Model file for the job. Use its own axes, mm. A direction names the side the tool comes from. Round coordinates to 2 decimals unless told otherwise and drop trailing zeros. Loops run counter-clockwise (first coordinate to the right, second up) from the corner with the lowest first, then second, coordinate; pieces in that order, holes last. Notation, with made-up numbers: (-9, 87.25) -> (14, 87.25) arc R19 ccw to (14, 98.25) -> close; hole circle Ø6 at (59.25, -17). An arc over 180 degrees is marked (long way). Use a Markdown table: item, result.
from build123d import *

# Parameters (mm, degrees)
BOSS_EXTRU_1_DEPTH      = 132
ESQUISSE2_W             = 78
ESQUISSE2_H             = 14.57
ENL_V_MAT_EXTRU_1_DEPTH = 132
ESQUISSE3_W             = 4.94012132
ESQUISSE3_H             = 29.556292602
ENL_V_MAT_EXTRU_2_DEPTH = 4
ESQUISSE4_R             = 1.3
ENL_V_MAT_EXTRU_3_DEPTH = 18
ESQUISSE6_R             = 2.9
ENL_V_MAT_EXTRU_5_DEPTH = 3


with BuildPart() as part:
    # Esquisse1 → Boss.-Extru.1 (new body)
    with BuildSketch(Plane.XY):
        with BuildLine():
            Line((-12.560062385, 0), (-18.560062385, 0))
            Line((-18.560062385, 0), (-18.560062385, 18))
            Line((-18.560062385, 18), (18.560062385, 18))
            Line((18.560062385, 18), (18.560062385, 0))
            Line((18.560062385, 0), (12.560062385, 0))
            ThreePointArc((12.560062385, 0), (0, 12.560062385), (-12.560062385, 0))
        make_face()
    extrude(amount=BOSS_EXTRU_1_DEPTH)

    # Esquisse2 → Enlèv. mat.-Extru.1 (cut)
    with BuildSketch(Plane.ZY.offset(18.560062385)):
        with Locations((66, 7.285)):
            Rectangle(ESQUISSE2_W, ESQUISSE2_H)
    extrude(amount=-ENL_V_MAT_EXTRU_1_DEPTH, mode=Mode.SUBTRACT)

    # Esquisse3 → Enlèv. mat.-Extru.2 (cut)
    with BuildSketch(Plane.XZ.offset(-14.57)):
        with Locations((0, 66)):
            Rectangle(ESQUISSE3_W, ESQUISSE3_H)
    extrude(amount=-ENL_V_MAT_EXTRU_2_DEPTH, mode=Mode.SUBTRACT)

    # Esquisse4 → Enlèv. mat.-Extru.3 (cut)
    with BuildSketch(Plane(origin=(0, 18, 0), x_dir=(1, 0, 0), z_dir=(0, 1, 0))):
        with Locations((15.560062385, -3)):
            Circle(ESQUISSE4_R)
        with Locations((15.560062385, -24)):
            Circle(ESQUISSE4_R)
        with Locations((-15.560062385, -3)):
            Circle(ESQUISSE4_R)
        with Locations((-15.560062385, -24)):
            Circle(ESQUISSE4_R)
        with Locations((-15.560062385, -108)):
            Circle(ESQUISSE4_R)
        with Locations((-15.560062385, -129)):
            Circle(ESQUISSE4_R)
        with Locations((15.560062385, -108)):
            Circle(ESQUISSE4_R)
        with Locations((15.560062385, -129)):
            Circle(ESQUISSE4_R)
    extrude(amount=-ENL_V_MAT_EXTRU_3_DEPTH, mode=Mode.SUBTRACT)

    # Esquisse6 → Enlèv. mat.-Extru.5 (cut)
    with BuildSketch(Plane(origin=(0, 18, 0), x_dir=(1, 0, 0), z_dir=(0, 1, 0))):
        with Locations((15.560062385, -3)):
            Circle(ESQUISSE6_R)
        with Locations((15.560062385, -24)):
            Circle(ESQUISSE6_R)
        with Locations((-15.560062385, -3)):
            Circle(ESQUISSE6_R)
        with Locations((-15.560062385, -24)):
            Circle(ESQUISSE6_R)
        with Locations((-15.560062385, -108)):
            Circle(ESQUISSE6_R)
        with Locations((-15.560062385, -129)):
            Circle(ESQUISSE6_R)
        with Locations((15.560062385, -108)):
            Circle(ESQUISSE6_R)
        with Locations((15.560062385, -129)):
            Circle(ESQUISSE6_R)
    extrude(amount=-ENL_V_MAT_EXTRU_5_DEPTH, mode=Mode.SUBTRACT)


solid = part.part
Q1. Flat gauge pins, fed straight in: pin 1 (1.6 mm diameter, centred on x = 15.56, z = 24, fed in from +Y); pin 2 (3 mm diameter, centred on x = -15.5, z = 2, fed in from +Y). Where does each tip first touch, or does it go through?
Results list:
| item | result |
|---|---|
| pin 1 | passes through |
| pin 2 | stops at y = 15 |
Q2. Tool access for faces 1 (the face through (-4.4, 12, 105)), 2 (the face through (-16.19, 16.52, 110.83)), 3 (the face through (2.47, 16, 66)): list every direction of +Z, -Z, +X, -X, +Y, -Y with a clear straight run to the whole face (end or side of a thin tool).
Results list:
| item | result |
|---|---|
| face 1 | +X, -X, -Y |
| face 2 | +Y |
| face 3 | +Y, -Y |
Q3. Band-saw the part on A-A, the plane z = 108. Give the cut face in (x, y), plus the area to 3 significant figures.
Results list:
| item | result |
|---|---|
| outline | (-18.56, 0) -> (-16.86, 0) -> (-16.86, 15) -> (-18.46, 15) -> (-18.46, 18) -> (-18.56, 18) -> close; (-14.26, 0) -> (-12.56, 0) arc R12.56 cw to (12.56, 0) -> (14.26, 0) -> (14.26, 15) -> (12.66, 15) -> (12.66, 18) -> (-12.66, 18) -> (-12.66, 15) -> (-14.26, 15) -> close; (16.86, 0) -> (18.56, 0) -> (18.56, 18) -> (18.46, 18) -> (18.46, 15) -> (16.86, 15) -> close |
| area | 308 mm² |
Q4. Pull direction Z, two halves, no side cores. Call faces 4 (the face through (0.276, 12.557, 118.311)), 5 (the face through (-15.73, 7.6, 127.71)): released by +Z, released by -Z, zero draft, split by the parting line, or undercut.
Results list:
| item | result |
|---|---|
| face 4 | zero draft |
| face 5 | undercut |
Q5. Band-saw the part on C-C, the plane z = 55. Give the cut face in (x, y).
Results list:
| item | result |
|---|---|
| outline | (-18.56, 14.57) -> (-2.47, 14.57) -> (-2.47, 18) -> (-18.56, 18) -> close; (2.47, 14.57) -> (18.56, 14.57) -> (18.56, 18) -> (2.47, 18) -> close |
Q6. Drill centre lines: L1, parallel to Z at x = -17, y = 7.5; L2, parallel to Z at x = 1, y = 17; L3, parallel to Y at x = 7.5, z = 48. Where is each one in solid material? Low to high. Write a range as from..to.
Results list:
| item | result |
|---|---|
| L1 | z = 0..27, 105..132 |
| L2 | z = 0..51.22, 80.78..132 |
| L3 | y = 14.57..18 |
Q7. Band-saw the part on B-B, the plane y = 6.5. Give the number of separate pieces and of enclosed holes in the cut face, plus the area to 3 significant figures.
Results list:
| item | result |
|---|---|
| separate pieces | 4 |
| enclosed holes | 8 |
| area | 801 mm² |
